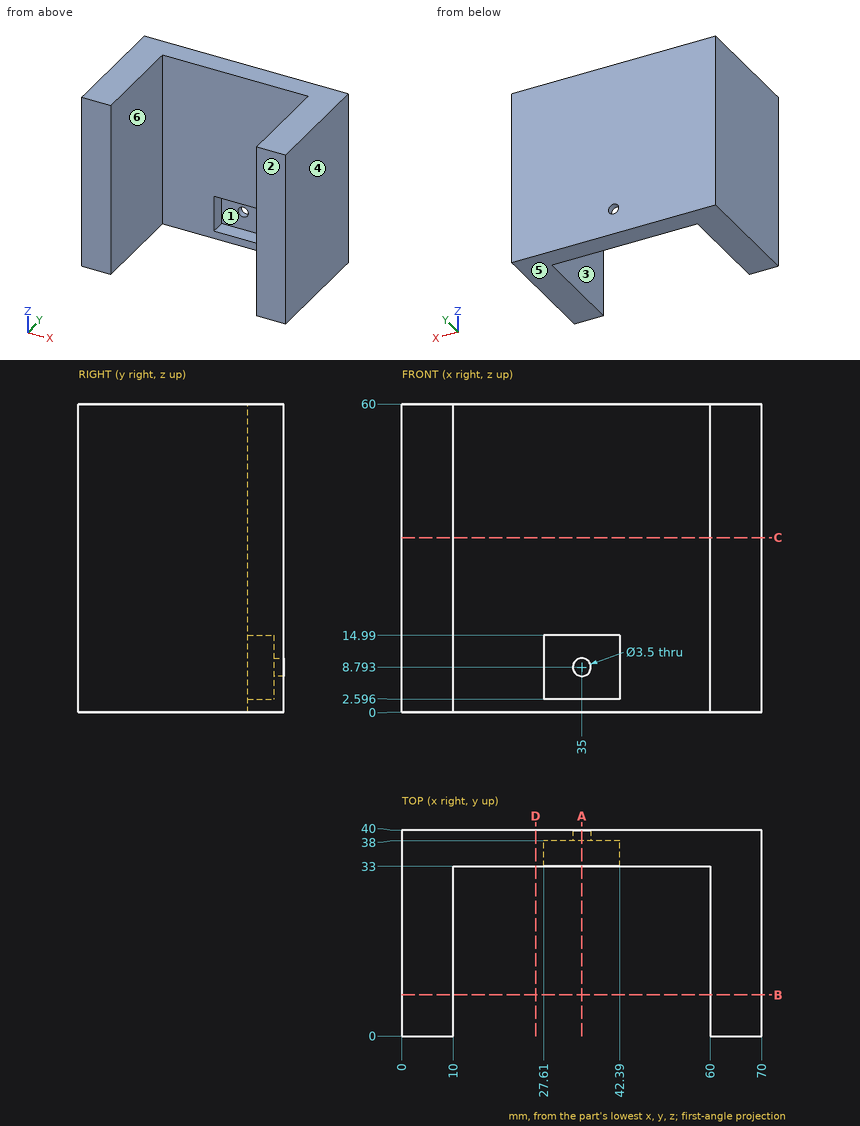
Design review of the part shown in the three views and the two pictorial views. Dimensions are in mm from the part's minimum x, y and z. A direction names the side the tool comes from. Round coordinates to 2 decimals unless told otherwise and drop trailing zeros. Write each loop counter-clockwise with the first axis right and the second up, starting at its lowest first coordinate (ties: lowest second). Pieces come first, ordered by that corner, then holes. Notation, with made-up numbers: (85.5, 69.5) -> (134.5, 69.5) arc R16 ccw to (134.5, 94.5) -> close; hole circle Ø8 at (-17.75, 20.5). An arc over 180 degrees is marked (long way). One line per question, with ' | ' between items. Start each with the question number.
1) Add section D-D (x = 26). Write out the cut boundary in (y, z), and give its area (3 significant figures).
2) Add section B-B (y = 8). Write out the cut boundary in (x, z).
3) Add section A-A (x = 35). Write out the cut boundary in (y, z) (1 decimal), and give its area (3 significant figures).
4) Machinability: for the marked faces 1, 2 and 3, which of the approach directions +Z, -Z, +X, -X, +Y, -Y give a long, thin tool a straight path to every point of the face, cutting with its end or side? Answer none if there is none.
5) Mouldability with a two-part tool opening along X and no side actions: class the marked faces 4, 5 and 6 as +X half, -X half, draft (parallel to the pull), parting line (faces both ways), or undercut.
6) Wall thickness on line 1 along X through (y, z) = (29, 20.5); line 2 along Z through (x, y) = (35, 39.05); line 3 along Y through (x, z) = (19, 22): over which ranges is each line inside the solid? List them lowest first.
7) Add section C-C (z = 34). Write out the cut boundary in (x, y), and give its area (3 significant figures).
8) For pin 1 Ø3.5 at (x, z) = (33, 11.5) entering from -Y; pin 2 Ø10 at (x, y) = (51.5, 8) entering from +Z; pin 3 Ø6 at (x, z) = (19.5, 14.5) entering from -Y, all flat-tipped, find the tip position at first contact; note any pin that passes through.
Reported:
1) outline: (33, 0) -> (40, 0) -> (40, 60) -> (33, 60) -> close | area: 420 mm²
2) outline: (0, 0) -> (10, 0) -> (10, 60) -> (0, 60) -> close; (60, 0) -> (70, 0) -> (70, 60) -> (60, 60) -> close
3) outline: (33, 0) -> (40, 0) -> (40, 7) -> (38, 7) -> (38, 2.6) -> (33, 2.6) -> close; (33, 15) -> (38, 15) -> (38, 10.5) -> (40, 10.5) -> (40, 60) -> (33, 60) -> close | area: 351 mm²
4) face 1: -Y | face 2: +Z, -Z, +X, -X, -Y | face 3: +Z, -Z, -Y
5) face 4: +X half | face 5: draft | face 6: undercut
6) line 1: x = 0 to 10, 60 to 70 | line 2: z = 0 to 7.04, 10.54 to 60 | line 3: y = 33 to 40
7) outline: (0, 0) -> (10, 0) -> (10, 33) -> (60, 33) -> (60, 0) -> (70, 0) -> (70, 40) -> (0, 40) -> close | area: 1,150 mm²
8) pin 1: stops at y = 38 | pin 2: passes through | pin 3: stops at y = 33
